```python
from build123d import *

# Parameters (mm, degrees)
F1_DEPTH = 2.9972
F2_D     = 4.4958
F3_D     = 16.66748
F4_D     = 8.4328
F5_D     = 6.5278


with BuildPart() as f1:
    # F0 (on Top) → F1 (new body)
    with BuildSketch(Plane.XY):
        with BuildLine():
            ThreePointArc((196.85, 60.96), (193.1302561211, 69.9402561211), (184.15, 73.66))
            Line((184.15, 73.66), (-184.15, 73.66))
            ThreePointArc((-184.15, 73.66), (-193.1302561211, 69.9402561211), (-196.85, 60.96))
            Line((-196.85, 60.96), (-196.85, -60.96))
            ThreePointArc((-196.85, -60.96), (-193.1302561211, -69.9402561211), (-184.15, -73.66))
            Line((-184.15, -73.66), (184.15, -73.66))
            ThreePointArc((184.15, -73.66), (193.1302561211, -69.9402561211), (196.85, -60.96))
            Line((196.85, -60.96), (196.85, 60.96))
        make_face()
    extrude(amount=F1_DEPTH)

    # F2 (through all)
    with Locations(Plane(origin=(0, 0, 0), x_dir=(1, 0, 0), z_dir=(0, 0, -1))):
        with Locations((165.1, -48.26), (73.66, -48.26), (50.8, -48.26), (-165.1, -48.26), (-184.15, -60.96), (-184.15, 60.96), (184.15, 60.96), (184.15, -60.96)):
            Hole(F2_D / 2)

    # F3 (through all)
    with Locations(Plane(origin=(0, 0, 0), x_dir=(1, 0, 0), z_dir=(0, 0, -1))):
        with Locations((20.955, -48.26), (-136.525, -48.26)):
            Hole(F3_D / 2)

    # F4 (through all)
    with Locations(Plane(origin=(0, 0, 0), x_dir=(1, 0, 0), z_dir=(0, 0, -1))):
        with Locations((165.1, 1.27), (73.66, 0), (20.955, 0), (-88.9, 0), (139.7, 44.45), (-88.9, 44.45), (-165.1, 0), (119.38, -22.86), (-12.7, 44.45)):
            Hole(F4_D / 2)

    # F5 (through all)
    with Locations(Plane(origin=(0, 0, 0), x_dir=(1, 0, 0), z_dir=(0, 0, -1))):
        with Locations((38.1, 44.45), (88.9, 44.45)):
            Hole(F5_D / 2)


solid = f1.part
```
For this review, take the finished solid that the model builds, in its own axes (mm). Round coordinates to 2 decimals unless told otherwise and drop trailing zeros. Loops run counter-clockwise (first coordinate to the right, second up) from the corner with the lowest first, then second, coordinate; pieces in that order, holes last.
(1) We need section B-B (x = 119.38). Give the boundary of the cut face in (y, z), plus the area to 3 significant figures.
Returned:
outline: (-73.66, 0) - (18.64, 0) - (18.64, 3) - (-73.66, 3) - close; (27.08, 0) - (73.66, 0) - (73.66, 3) - (27.08, 3) - close
area: 416 mm2
(2) We need section A-A (y = 22.86). Give the boundary of the cut face in (x, z), plus the area to 3 significant figures.
Returned:
outline: (-196.85, 0) - (115.16, 0) - (115.16, 3) - (-196.85, 3) - close; (123.6, 0) - (196.85, 0) - (196.85, 3) - (123.6, 3) - close
area: 1,150 mm2
(3) We need section C-C (z = 0.55). State how many separate pieces and enclosed holes the cut face has, plus the area to 3 significant figures.
Returned:
separate pieces: 1
enclosed holes: 21
area: 56,700 mm2
(4) Mouldability with a two-part tool opening along Y and no side actions: class faces 1 (the flat face through (-3, 1, 0)), 2 (the cylindrical face through (-12.15, -48.63, 1.52)), 3 (the cylindrical face through (193.23, 69.84, 1.48)) as released by +Y, released by -Y, zero draft, split by the parting line, or undercut.
Returned:
face 1: zero draft
face 2: undercut
face 3: released by +Y
(5) Wall thickness on line 1 along X through (y, z) = (-44.45, 0.9); line 2 along Y through (x, z) = (184.15, 0.6); line 3 along Y through (x, z) = (165.1, 0.9): over which ranges is each line inside the solid? List them lowest first.
Returned:
line 1: x = -196.85 to -93.12, -84.68 to -16.92, -8.48 to 34.84, 41.36 to 85.64, 92.16 to 135.48, 143.92 to 196.85
line 2: y = -73.66 to -63.21, -58.71 to 58.71, 63.21 to 73.66
line 3: y = -73.66 to -5.49, 2.95 to 46.01, 50.51 to 73.66
(6) Clearance check with a flat-ended pin moving along its axis: P1, Ø4, axis at x = -108, y = 53, coming from the -Z side. State where the tip first meets the part, or that it passes through.
Returned:
P1: stops at z = 0
